Here's how the part is built. I have some questions about the finished solid (model axes, mm). A direction names the side the tool comes from. Give positions to 0.01 mm unless a question says otherwise; leave off trailing zeros. Write each loop counter-clockwise with the first axis right and the second up, starting at its lowest first coordinate (ties: lowest second). Pieces come first, ordered by that corner, then holes. Notation, with made-up numbers: (-31, 36.25) -> (-22, 36.25) arc R20 ccw to (-22, 58.25) -> close; hole circle Ø11 at (-13.75, -35.75). An arc over 180 degrees is marked (long way). Put each result on its own line as item: value. Start each with the question number.
from build123d import *

# Parameters (mm, degrees)
SKETCH2_R           = 1.6
SKETCH2_R_2         = 13
SKETCH2_R_3         = 2.75
BOSS_EXTRUDE1_DEPTH = 5


with BuildPart() as part:
    # Sketch2 → Boss-Extrude1 (new body)
    with BuildSketch(Plane(origin=(0, 0, 0), x_dir=(1, 0, 0), z_dir=(0, 1, 0))):
        Polygon((0, 0), (20, 0), (20, 17), (63, 17), (63, 60), (80, 60), (80, 80), (0, 80), align=None)
        with Locations((57, 23)):
            Circle(SKETCH2_R, mode=Mode.SUBTRACT)
        with Locations((57, 54)):
            Circle(SKETCH2_R, mode=Mode.SUBTRACT)
        with Locations((26, 23)):
            Circle(SKETCH2_R, mode=Mode.SUBTRACT)
        with Locations((26, 54)):
            Circle(SKETCH2_R, mode=Mode.SUBTRACT)
        with Locations((41.5, 38.5)):
            Circle(SKETCH2_R_2, mode=Mode.SUBTRACT)
        with Locations((10, 8)):
            Circle(SKETCH2_R_3, mode=Mode.SUBTRACT)
        with Locations((72, 70)):
            Circle(SKETCH2_R_3, mode=Mode.SUBTRACT)
        with Locations((41.5, 70)):
            Circle(SKETCH2_R_3, mode=Mode.SUBTRACT)
        with Locations((10, 38.5)):
            Circle(SKETCH2_R_3, mode=Mode.SUBTRACT)
    extrude(amount=BOSS_EXTRUDE1_DEPTH)


solid = part.part
1) I want a section at A-A, the plane z = -8. Write out the boundary of the cut face in (x, y).
2) I need wall thicknesses on probe 1 along X at (y, z) = (1.1, -23); probe 2 along X at (y, z) = (3.8, -70); probe 3 along X at (y, z) = (2.5, -8). Which ranges of each line are inside material? Lowest first, please.
3) I want a section at B-B, the plane x = 57. Write out the boundary of the cut face in (y, z), and give its area (3 significant figures).
4) Which directions (+Z, -Z, +X, -X, +Y, -Y) give clear straight access to the entire face, cutting with the end or side of a thin tool? Please do faces 1 (the flat face through (41, 2, -17)), 2 (the flat face through (80, 2, -70)).
5) I want a section at C-C, the plane z = -38.5. Write out the boundary of the cut face in (x, y), and give its area (4 significant figures).
6) Thinking about a two-plate mould opening in Z: for faces 3 (the cylindrical face through (58.526, 2.465, -23.481)), 4 (the flat face through (41, 2, -80)), 5 (the cylindrical face through (25.792, 2.465, -24.586)), 6 (the flat face through (0, 2, -41)), which applies, released by +Z, released by -Z, zero draft, split by the parting line, or undercut?
7) I'm going to push flat-ended pins straight in: pin 1 Ø1.5 at (x, y) = (25, 2.5) entering from +Z; pin 2 Ø1.5 at (y, z) = (2.5, -45.5) entering from +X. Where does each tip first touch, or does it pass through?
8) I want a section at D-D, the plane y = 1.95. State how many separate pieces and enclosed holes the cut face has, and give its area (3 significant figures).
Established:
1. outline: (0, 0) -> (7.25, 0) -> (7.25, 5) -> (0, 5) -> close; (12.75, 0) -> (20, 0) -> (20, 5) -> (12.75, 5) -> close
2. probe 1: x = 0 to 24.4, 27.6 to 55.4, 58.6 to 63
2. probe 2: x = 0 to 38.75, 44.25 to 69.25, 74.75 to 80
2. probe 3: x = 0 to 7.25, 12.75 to 20
3. outline: (0, -80) -> (5, -80) -> (5, -55.6) -> (0, -55.6) -> close; (0, -52.4) -> (5, -52.4) -> (5, -24.6) -> (0, -24.6) -> close; (0, -21.4) -> (5, -21.4) -> (5, -17) -> (0, -17) -> close
3. area: 283 mm2
4. face 1: +Z, +X, +Y, -Y
4. face 2: +Z, -Z, +X, +Y, -Y
5. outline: (0, 0) -> (7.25, 0) -> (7.25, 5) -> (0, 5) -> close; (12.75, 0) -> (28.5, 0) -> (28.5, 5) -> (12.75, 5) -> close; (54.5, 0) -> (63, 0) -> (63, 5) -> (54.5, 5) -> close
5. area: 157.5 mm2
6. face 3: undercut
6. face 4: released by -Z
6. face 5: undercut
6. face 6: zero draft
7. pin 1: stops at z = -17
7. pin 2: stops at x = 63
8. separate pieces: 1
8. enclosed holes: 9
8. area: 3,990 mm2
